Part model, mm, in its own coordinate system. A direction names the side the tool comes from. Coordinates: 2 decimals unless noted, no trailing zeros. Loops run counter-clockwise (first coordinate to the right, second up) from the corner with the lowest first, then second, coordinate; pieces in that order, holes last. Notation, with made-up numbers: (29.25, -21.5) - (37.25, -21.5) arc R31 ccw to (37.25, 11.5) - close; hole circle Ø6 at (52.25, 70.5). An arc over 180 degrees is marked (long way). Use a Markdown table: item, result. Add a question column.
1. Band-saw the part on A-A, the plane z = 0. Give the cut face in (x, y).
2. Wall check: probe 1 along X at (y, z) = (14, 12); probe 2 along X at (y, z) = (13.35, 0); probe 3 along X at (y, z) = (7.75, 0). Give the ranges that are in metal, low to high. Write a range as [from, to].
3. Pull direction Z, two halves, no side cores. Call faces 1 (the flat face through (0, 14, 24)), 2 (the cylindrical face through (-17.61, 14.67, -10.76)), 3 (the flat face through (0, 16, -2)): pulls with the +Z half, pulls with the -Z half, needs draft (parallel to the pull), parting line crosses it, or undercut.
4. Drop flat-ended pins along their axis: pin 1 (3 mm diameter, centred on y = 8, z = 1.5, fed in from +X); pin 2 (4 mm diameter, centred on y = 10, z = 27, fed in from +X); pin 3 (3 mm diameter, centred on x = 18, z = -12, fed in from -Y); pin 4 (6 mm diameter, centred on x = 6, y = 3.5, fed in from +Z). Give the stop position or say it passes through.
5. 3-axis set-ups, long thin cutter, end or side, ignore diameter. For faces 4 (the flat face through (0, 11.5, -1)), 5 (the cylindrical face through (1.539, 7.888, -34.966)), 6 (the flat face through (-18, 13.5, 12)): which of +Z, -Z, +X, -X, +Y, -Y reach the whole face in a straight line?
6. Band-saw the part on D-D, the plane z = 25. Give the cut face in (x, y), plus the area to 3 significant figures.
7. Band-saw the part on C-C, the plane y = 4. Give the cut face in (x, z).
8. Band-saw the part on B-B, the plane x = 0. Give the cut face in (y, z).
from build123d import *

# Parameters (mm, degrees)
SKETCH_1_R          = 35
EXTRUDE_1_DEPTH     = 16
SKETCH_2_R          = 34
CUT_EXTRUDE_1_DEPTH = 11.5
SKETCH_3_R          = 1.25
CUT_EXTRUDE_4_DEPTH = 16
CUT_EXTRUDE_START   = -9
CUT_EXTRUDE_5_DEPTH = 9
SKETCH_5_R          = 1.3
CUT_EXTRUDE_6_DEPTH = 2.5
CHAMFER_1_SIZE      = 0.2


with BuildPart() as part:
    # 草圖1 → 填料-伸長1 (new body)
    with BuildSketch(Plane(origin=(0, 0, 0), x_dir=(1, 0, 0), z_dir=(0, 1, 0))):
        with Locations(Location((0, 0, 0), (0, 0, 270))):
            Circle(SKETCH_1_R)
    extrude(amount=EXTRUDE_1_DEPTH)

    # 草圖2 → 除料-伸長1 (cut)
    with BuildSketch(Plane.XZ):
        with Locations(Location((0, 0, 0), (0, 0, 270))):
            Circle(SKETCH_2_R)
    extrude(amount=-CUT_EXTRUDE_1_DEPTH, mode=Mode.SUBTRACT)

    # 草圖3 → 除料-伸長4 (cut)
    with BuildSketch(Plane(origin=(0, 0, 0), x_dir=(1, 0, 0), z_dir=(0, 1, 0))):
        with Locations(Location((-31.25, 0, 0), (0, 0, 90))):
            Circle(SKETCH_3_R)
        with Locations(Location((31.25, 0, 0), (0, 0, 90))):
            Circle(SKETCH_3_R)
    extrude(amount=CUT_EXTRUDE_4_DEPTH, mode=Mode.SUBTRACT)

    # 草圖4 → 除料-伸長5 (cut)
    with BuildSketch(Plane(origin=(0, 16, 0), x_dir=(1, 0, 0), z_dir=(0, 1, 0)).offset(CUT_EXTRUDE_START)):
        with BuildLine():
            Line((-14, -24), (14, -24))
            Line((14, -24), (14, -32.078029865))
            ThreePointArc((14, -32.078029865), (0, -35), (-14, -32.078029865))
            Line((-14, -32.078029865), (-14, -24))
        make_face()
    extrude(amount=CUT_EXTRUDE_5_DEPTH, mode=Mode.SUBTRACT)

    # 草圖5 → 除料-伸長6 (cut)
    with BuildSketch(Plane(origin=(0, 16, 0), x_dir=(1, 0, 0), z_dir=(0, 1, 0))):
        with Locations(Location((-18, 12, 0), (0, 0, 270))):
            Circle(SKETCH_5_R)
        with Locations(Location((18, 12, 0), (0, 0, 270))):
            Circle(SKETCH_5_R)
        with Locations(Location((18, -12, 0), (0, 0, 270))):
            Circle(SKETCH_5_R)
        with Locations(Location((-18, -12, 0), (0, 0, 270))):
            Circle(SKETCH_5_R)
    extrude(amount=-CUT_EXTRUDE_6_DEPTH, mode=Mode.SUBTRACT)

    # 導角1
    chamfer_1_edges = [part.edges().sort_by_distance(p)[0] for p in [
        (-18, 16, 10.7),
        (18, 16, 10.7),
        (18, 16, -13.3),
        (-18, 16, -13.3),
    ]]
    chamfer(chamfer_1_edges, length=CHAMFER_1_SIZE)


solid = part.part
Geometry check:
| question | item | result |
|---|---|---|
| 1 | outline | (-35, 0) - (-34, 0) - (-34, 11.5) - (-32.5, 11.5) - (-32.5, 16) - (-35, 16) - close; (-30, 11.5) - (30, 11.5) - (30, 16) - (-30, 16) - close; (32.5, 11.5) - (34, 11.5) - (34, 0) - (35, 0) - (35, 16) - (32.5, 16) - close |
| 2 | probe 1 | x = [-32.88, -19.3], [-16.7, 16.7], [19.3, 32.88] |
| 2 | probe 2 | x = [-35, -32.5], [-30, 30], [32.5, 35] |
| 2 | probe 3 | x = [-35, -34], [34, 35] |
| 3 | face 1 | pulls with the +Z half |
| 3 | face 2 | undercut |
| 3 | face 3 | needs draft |
| 4 | pin 1 | stops at x = 35 |
| 4 | pin 2 | stops at x = 24.49 |
| 4 | pin 3 | stops at y = 11.5 |
| 4 | pin 4 | stops at z = 34.87 |
| 5 | face 4 | -Y |
| 5 | face 5 | +Y, -Y |
| 5 | face 6 | +Y |
| 6 | outline | (-24.49, 0) - (-23.04, 0) - (-23.04, 11.5) - (-14, 11.5) - (-14, 16) - (-24.49, 16) - close; (14, 11.5) - (23.04, 11.5) - (23.04, 0) - (24.49, 0) - (24.49, 16) - (14, 16) - close |
| 6 | area | 128 mm^2 |
| 7 | outline | circle Ø70 at (0, 0); hole circle Ø68 at (0, 0) |
| 8 | outline | (0, -35) - (16, -35) - (16, 24) - (11.5, 24) - (11.5, -34) - (0, -34) - close; (0, 34) - (7, 34) - (7, 35) - (0, 35) - close |
